from build123d import *

# Parameters (mm, degrees)
CROQUIS1_R              = 21
SALIENTE_EXTRUIR1_DEPTH = 68
CROQUIS2_R              = 11
SALIENTE_EXTRUIR2_DEPTH = 2.5
CROQUIS3_R              = 3
SALIENTE_EXTRUIR3_DEPTH = 25.6
CROQUIS4_W              = 20
CROQUIS4_H              = 8.467586068
SALIENTE_EXTRUIR4_DEPTH = 5
CROQUIS6_W              = 20
CROQUIS6_H              = 8.467586068
SALIENTE_EXTRUIR5_DEPTH = 5
CORTAR_EXTRUIR1_DEPTH   = 103.753459728
CROQUIS8_R              = 1.5
CORTAR_EXTRUIR2_DEPTH   = 10


with BuildPart() as part:
    # Croquis1 → Saliente-Extruir1 (new body)
    with BuildSketch(Plane.XY):
        Circle(CROQUIS1_R)
    extrude(amount=SALIENTE_EXTRUIR1_DEPTH)

    # Croquis2 → Saliente-Extruir2 (add)
    with BuildSketch(Plane.XY.offset(68)):
        Circle(CROQUIS2_R)
    extrude(amount=SALIENTE_EXTRUIR2_DEPTH)

    # Croquis3 → Saliente-Extruir3 (add)
    with BuildSketch(Plane.XY.offset(70.5)):
        Circle(CROQUIS3_R)
    extrude(amount=SALIENTE_EXTRUIR3_DEPTH)

    # Croquis4 → Saliente-Extruir4 (add, symmetric)
    with BuildSketch(Plane(origin=(21, 0, 0), x_dir=(0, 0, -1), z_dir=(1, 0, 0))):
        with Locations((5, 0.203649565)):
            Rectangle(CROQUIS4_W, CROQUIS4_H)
    extrude(amount=SALIENTE_EXTRUIR4_DEPTH, both=True)

    # Croquis6 → Saliente-Extruir5 (add, symmetric)
    with BuildSketch(Plane(origin=(-21, 0, 0), x_dir=(0, 0, -1), z_dir=(1, 0, 0))):
        with Locations((5, 0.203649565)):
            Rectangle(CROQUIS6_W, CROQUIS6_H)
    extrude(amount=SALIENTE_EXTRUIR5_DEPTH, both=True)

    # Croquis7 → Cortar-Extruir1 (cut, through all)
    with BuildSketch(Plane(origin=(0, 4.437442599, 0), x_dir=(1, 0, 0), z_dir=(0, 1, 0))):
        Polygon((16, 3.735002253), (21, 3.735002253), (21, 15), (-21, 15), (-21, 3.735002253), align=None)
    extrude(amount=-CORTAR_EXTRUIR1_DEPTH, mode=Mode.SUBTRACT)

    # Croquis8 → Cortar-Extruir2 (cut)
    with BuildSketch(Plane.XY.offset(68)):
        with Locations((-16, 0)):
            Circle(CROQUIS8_R)
        with Locations((16, 0)):
            Circle(CROQUIS8_R)
    extrude(amount=-CORTAR_EXTRUIR2_DEPTH, mode=Mode.SUBTRACT)


solid = part.part
Build history of the part. All positions in model axes, mm. A direction names the side the tool comes from. Coordinates: 2 decimals unless noted, no trailing zeros. Order: outer loops, then holes, each group sorted by start corner. A loop starts at its lowest first (then second) coordinate and runs counter-clockwise, first axis right, second up. Notation, with made-up numbers: (88, -6) - (112, -6) arc R18 ccw to (112, 27) - close; hole circle Ø7 at (18, 16.25). An arc over 180 degrees is marked (long way). Write item = value, one per line. Start each with the question number.
1) Flat gauge pins, fed straight in: pin 1 Ø5 at (x, z) = (-4.5, 38) entering from +Y; pin 2 Ø4 at (x, y) = (7.5, 7) entering from -Z; pin 3 Ø21 at (x, y) = (3, 0.5) entering from +Z; pin 4 Ø3 at (y, z) = (15, 9) entering from +X. Where does each tip first touch, or does it go through?
2) Saw through at C-C on z = 72. Write the cut outline in (x, y), then the cut area to 3 significant figures.
3) Two-plate mould, pull along Y, no slides. Class faces 1 (the face through (-2.38, -10.74, 69.23)), 2 (the face through (-16, 0, 58)), 3 (the face through (-23, 0, 5)), 4 (the face through (14.5, 0.07, 63.07)): pulls with the +Y half, pulls with the -Y half, needs draft (parallel to the pull), parting line crosses it, or undercut.
4) Saw through at A-A on x = 0. Write the cut outline in (y, z), then the cut area to 3 significant figures.
5) 3-axis set-ups, long thin cutter, end or side, ignore diameter. For faces 5 (the face through (-22, 4.437, -5)), 6 (the face through (22, -4.03, -5)), 7 (the face through (21, 0, -9)), 8 (the face through (-17.5, 0.07, 63.07)): which of +Z, -Z, +X, -X, +Y, -Y reach the whole face in a straight line?
6) Wall check: line 1 along Z through (x, y) = (4, 14.5); line 2 along Z through (x, y) = (3.5, 7.5); line 3 along Y through (x, z) = (16, 61). Give the ranges that are in metal, low to high. Write a range as from..to.
7) Saw through at D-D on x = -9. Write the cut outline in (y, z).
From the geometry:
q1.pin_1 = 20.9
q1.pin_2 = 0
q1.pin_3 = 96.1
q1.pin_4 = 16.09
q2.outline = circle Ø6 at (0, 0)
q2.area = 28.3 mm^2
q3.face_1 = parting line crosses it
q3.face_2 = undercut
q3.face_3 = needs draft
q3.face_4 = undercut
q4.outline = (-21, 0) - (21, 0) - (21, 68) - (11, 68) - (11, 70.5) - (3, 70.5) - (3, 96.1) - (-3, 96.1) - (-3, 70.5) - (-11, 70.5) - (-11, 68) - (-21, 68) - close
q4.area = 3,060 mm^2
q5.face_5 = -Z, -X, +Y
q5.face_6 = -Z, +X, -Y
q5.face_7 = -Z, +Y, -Y
q5.face_8 = +Z
q6.line_1 = 0..68
q6.line_2 = 0..70.5
q6.line_3 = -13.6..-1.5, 1.5..13.6
q7.outline = (-18.97, 0) - (18.97, 0) - (18.97, 68) - (6.32, 68) - (6.32, 70.5) - (-6.32, 70.5) - (-6.32, 68) - (-18.97, 68) - close
